Geometry check sheet. Reference: drawing and pictorial views, mm from the part's lowest x, y, z. A direction names the side the tool comes from. Give positions to 0.01 mm unless a question says otherwise; leave off trailing zeros. Write each loop counter-clockwise with the first axis right and the second up, starting at its lowest first coordinate (ties: lowest second). Pieces come first, ordered by that corner, then holes.
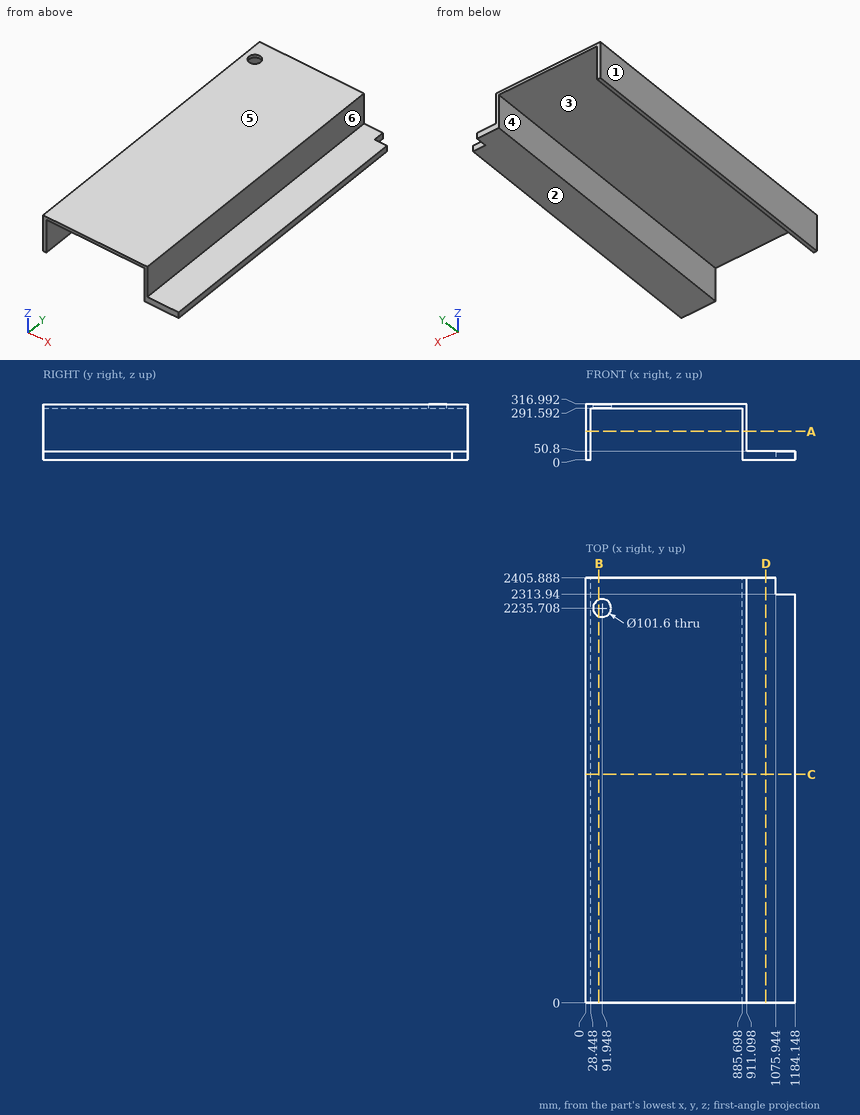
Item 1: Sectioned sample at D-D on x = 1019. Record the cut outline in (y, z).
Answer key:
outline: (0, 0) - (2405.89, 0) - (2405.89, 50.8) - (0, 50.8) - close
Item 2: Sectioned sample at A-A on z = 162. Record the cut outline in (x, y), then the cut area to 3 significant figures.
Answer key:
outline: (0, 0) - (28.45, 0) - (28.45, 2405.89) - (0, 2405.89) - close; (885.7, 0) - (911.1, 0) - (911.1, 2405.89) - (885.7, 2405.89) - close
area: 130,000 mm2
Item 3: Set-up check for the marked faces 4, 5 and 6: record each of +Z, -Z, +X, -X, +Y, -Y from which the full face is reachable in a straight line by a thin tool's end or side.
Answer key:
face 4: -Z, +Y, -Y
face 5: +Z, +X, -X, +Y, -Y
face 6: +Z, +X, +Y, -Y
Item 4: Release check for a two-part mould opening along X. For the marked faces 1, 2 and 3 record: released by +X, released by -X, zero draft, split by the parting line, or undercut.
Answer key:
face 1: released by -X
face 2: zero draft
face 3: undercut
Item 5: Sectioned sample at B-B on x = 73.5. Record the cut outline in (y, z).
Answer key:
outline: (0, 291.59) - (2188.38, 291.59) - (2188.38, 316.99) - (0, 316.99) - close; (2283.04, 291.59) - (2405.89, 291.59) - (2405.89, 316.99) - (2283.04, 316.99) - close
Item 6: Depth check by flat-ended pin: pin 1 (1.5 mm diameter, centred on y = 1416, z = 58.5, fed in from +X); pin 2 (15 mm diameter, centred on x = 1103, z = 15.5, fed in from +Y); pin 3 (6 mm diameter, centred on y = 2085, z = 72.5, fed in from -X). Enter the tip coordinate at first touch or a pass-through.
Answer key:
pin 1: stops at x = 911.1
pin 2: stops at y = 2313.94
pin 3: stops at x = 0
Item 7: Scan lines: line 1 along X through (y, z) = (2227, 154.5); line 2 along Z through (x, y) = (504, 1464); line 3 along Z through (x, y) = (1090.5, 121.5). Record each from-to range of solid material in increasing order.
Answer key:
line 1: x = 0 to 28.45, 885.7 to 911.1
line 2: z = 291.59 to 316.99
line 3: z = 0 to 50.8
Item 8: Sectioned sample at C-C on y = 1293.5. Record the cut outline in (x, z), then the cut area to 3 significant figures.
Answer key:
outline: (0, 0) - (28.45, 0) - (28.45, 291.59) - (885.7, 291.59) - (885.7, 0) - (1184.15, 0) - (1184.15, 50.8) - (911.1, 50.8) - (911.1, 316.99) - (0, 316.99) - close
area: 52,700 mm2
